Geometry check sheet. Reference: the model listing, model coordinates, mm. A direction names the side the tool comes from. Coordinates: 2 decimals unless noted, no trailing zeros. Loops run counter-clockwise (first coordinate to the right, second up) from the corner with the lowest first, then second, coordinate; pieces in that order, holes last. Notation, with made-up numbers: (76, 32) - (86, 32) arc R19 ccw to (86, 67) - close; hole circle Ø3 at (-20.5, 30.5). An arc over 180 degrees is marked (long way). One line per item, written item: value.
from build123d import *

# Parameters (mm, degrees)
SKETCH2_W           = 12
SKETCH2_H           = 12
BOSS_EXTRUDE1_DEPTH = 3.25
SKETCH3_R           = 3.37
SKETCH3_W           = 3.8
SKETCH3_H           = 3.8
SKETCH3_W_2         = 3
SKETCH3_H_2         = 3
BOSS_EXTRUDE2_DEPTH = 0.5
SKETCH3_4_W         = 3
SKETCH3_4_H         = 3
BOSS_EXTRUDE3_DEPTH = 4
BOSS_EXTRUDE4_START = 2
SKETCH3_5_W         = 3.8
SKETCH3_5_H         = 3.8
SKETCH3_5_W_2       = 3
SKETCH3_5_H_2       = 3
BOSS_EXTRUDE4_DEPTH = 2
SKETCH4_W           = 20
SKETCH4_H           = 17
SKETCH4_R           = 1
BOSS_EXTRUDE5_DEPTH = 3.5
BOSS_EXTRUDE6_START = 3
SKETCH7_R           = 5.85
BOSS_EXTRUDE6_DEPTH = 5.7


with BuildPart() as part:
    # Sketch2 → Boss-Extrude1 (new body)
    with BuildSketch(Plane(origin=(0, 0, 0), x_dir=(1, 0, 0), z_dir=(0, 1, 0))):
        Rectangle(SKETCH2_W, SKETCH2_H)
    extrude(amount=BOSS_EXTRUDE1_DEPTH)

    # Sketch3 → Boss-Extrude2 (add)
    # profile 1 of 2: a face of its own
    with BuildSketch(Plane(origin=(0, 3.25, 0), x_dir=(1, 0, 0), z_dir=(0, 1, 0))):
        with Locations(Location((0, 0, 0), (0, 0, 90))):
            Circle(SKETCH3_R)
        Rectangle(SKETCH3_W, SKETCH3_H, mode=Mode.SUBTRACT)
    # profile 2 of 2: a face of its own
    with BuildSketch(Plane(origin=(0, 3.25, 0), x_dir=(1, 0, 0), z_dir=(0, 1, 0))):
        Rectangle(SKETCH3_W, SKETCH3_H)
        Rectangle(SKETCH3_W_2, SKETCH3_H_2, mode=Mode.SUBTRACT)
    extrude(amount=BOSS_EXTRUDE2_DEPTH)

    # Sketch3_4 → Boss-Extrude3 (add)
    with BuildSketch(Plane(origin=(0, 3.25, 0), x_dir=(1, 0, 0), z_dir=(0, 1, 0))):
        Rectangle(SKETCH3_4_W, SKETCH3_4_H)
    extrude(amount=BOSS_EXTRUDE3_DEPTH)

    # Sketch3_5 → Boss-Extrude4 (add)
    with BuildSketch(Plane(origin=(0, 3.25, 0), x_dir=(1, 0, 0), z_dir=(0, 1, 0)).offset(BOSS_EXTRUDE4_START)):
        Rectangle(SKETCH3_5_W, SKETCH3_5_H)
        Rectangle(SKETCH3_5_W_2, SKETCH3_5_H_2, mode=Mode.SUBTRACT)
    extrude(amount=BOSS_EXTRUDE4_DEPTH)

    # Sketch4 → Boss-Extrude5 (add)
    with BuildSketch(Plane.XZ):
        with Locations((0, -2.5)):
            Rectangle(SKETCH4_W, SKETCH4_H)
        with Locations(Location((-7.8, -8.8, 0), (0, 0, 270))):
            Circle(SKETCH4_R, mode=Mode.SUBTRACT)
        with Locations(Location((7.8, -8.8, 0), (0, 0, 90))):
            Circle(SKETCH4_R, mode=Mode.SUBTRACT)
    extrude(amount=BOSS_EXTRUDE5_DEPTH)

    # Sketch7 → Boss-Extrude6 (add)
    with BuildSketch(Plane(origin=(0, 3.25, 0), x_dir=(1, 0, 0), z_dir=(0, 1, 0)).offset(BOSS_EXTRUDE6_START)):
        with Locations(Location((0, 0, 0), (0, 0, 270))):
            Circle(SKETCH7_R)
    extrude(amount=BOSS_EXTRUDE6_DEPTH)


solid = part.part
(1) Cross-section at D-D on z = 0. Record the cut outline in (x, y).
Reply:
outline: (-10, -3.5) - (10, -3.5) - (10, 0) - (6, 0) - (6, 3.25) - (3.37, 3.25) - (3.37, 3.75) - (1.5, 3.75) - (1.5, 5.25) - (1.9, 5.25) - (1.9, 6.25) - (5.85, 6.25) - (5.85, 11.95) - (-5.85, 11.95) - (-5.85, 6.25) - (-1.9, 6.25) - (-1.9, 5.25) - (-1.5, 5.25) - (-1.5, 3.75) - (-3.37, 3.75) - (-3.37, 3.25) - (-6, 3.25) - (-6, 0) - (-10, 0) - close
(2) Access from +Z, -Z, +X, -X, +Y, -Y to the whole of each face (thin tool, end or side, straight path). Record for faces 1 (the face through (0, 6, 1.9)), 2 (the face through (-5.19, 9.06, 2.7)), 3 (the face through (-1.9, 6, 0)).
Reply:
face 1: +Z, +X, -X
face 2: +Y
face 3: +Z, -Z, -X
(3) Material ranges on probe 1 along X at (y, z) = (-0.95, -8.8); probe 2 along Y at (x, z) = (0.25, -4.25); probe 3 along Z at (x, y) = (7.8, -1.8), recorded low to high. Write a range as from..to.
Reply:
probe 1: -10..-8.8, -6.8..6.8, 8.8..10
probe 2: -3.5..3.25, 6.25..11.95
probe 3: -11..-9.8, -7.8..6
(4) Cross-section at C-C on y = -0.5. Record the cut outline in (x, z), and give its area (3 significant figures).
Reply:
outline: (-10, -11) - (10, -11) - (10, 6) - (-10, 6) - close; hole circle Ø2 at (-7.8, -8.8); hole circle Ø2 at (7.8, -8.8)
area: 334 mm2
(5) Release check for a two-part mould opening along Y. For faces 4 (the face through (0, 11.95, 0)), 5 (the face through (1.7, 5.25, 0)), 6 (the face through (0, -3.5, -2)) record: pulls with the +Y half, pulls with the -Y half, needs draft (parallel to the pull), parting line crosses it, or undercut.
Reply:
face 4: pulls with the +Y half
face 5: undercut
face 6: pulls with the -Y half
(6) Cross-section at A-A on x = -7.8. Record the cut outline in (y, z).
Reply:
outline: (-3.5, -11) - (0, -11) - (0, -9.8) - (-3.5, -9.8) - close; (-3.5, -7.8) - (0, -7.8) - (0, 6) - (-3.5, 6) - close
(7) Go/stop test with flat-tipped pins: pin 1 Ø1.6 at (x, y) = (0.5, 4.5) entering from -Z; pin 2 Ø2 at (x, y) = (-5, 7.5) entering from +Z; pin 3 Ø0.8 at (x, y) = (0, 6) entering from -Z; pin 4 Ø3.5 at (y, z) = (1, 0) entering from +X. Record where each tip stops, or that it passes through.
Reply:
pin 1: z = -3.36
pin 2: z = 4.27
pin 3: z = -5.85
pin 4: x = 10
(8) Cross-section at B-B on z = -8.8. Record the cut outline in (x, y).
Reply:
outline: (-10, -3.5) - (-8.8, -3.5) - (-8.8, 0) - (-10, 0) - close; (-6.8, -3.5) - (6.8, -3.5) - (6.8, 0) - (-6.8, 0) - close; (8.8, -3.5) - (10, -3.5) - (10, 0) - (8.8, 0) - close
